Verification items for this drawing (mm, ordinates from the low corner). A direction names the side the tool comes from. Coordinates: 2 decimals unless noted, no trailing zeros. Loops run counter-clockwise (first coordinate to the right, second up) from the corner with the lowest first, then second, coordinate; pieces in that order, holes last. Notation, with made-up numbers: M 50,57.25 L 61,57.25 A12 cw 61,72.25 Z; hole C 54,12.5 d4. An arc over 180 degrees is marked long. Use CSV: the item, a comma, the result in double quotes.
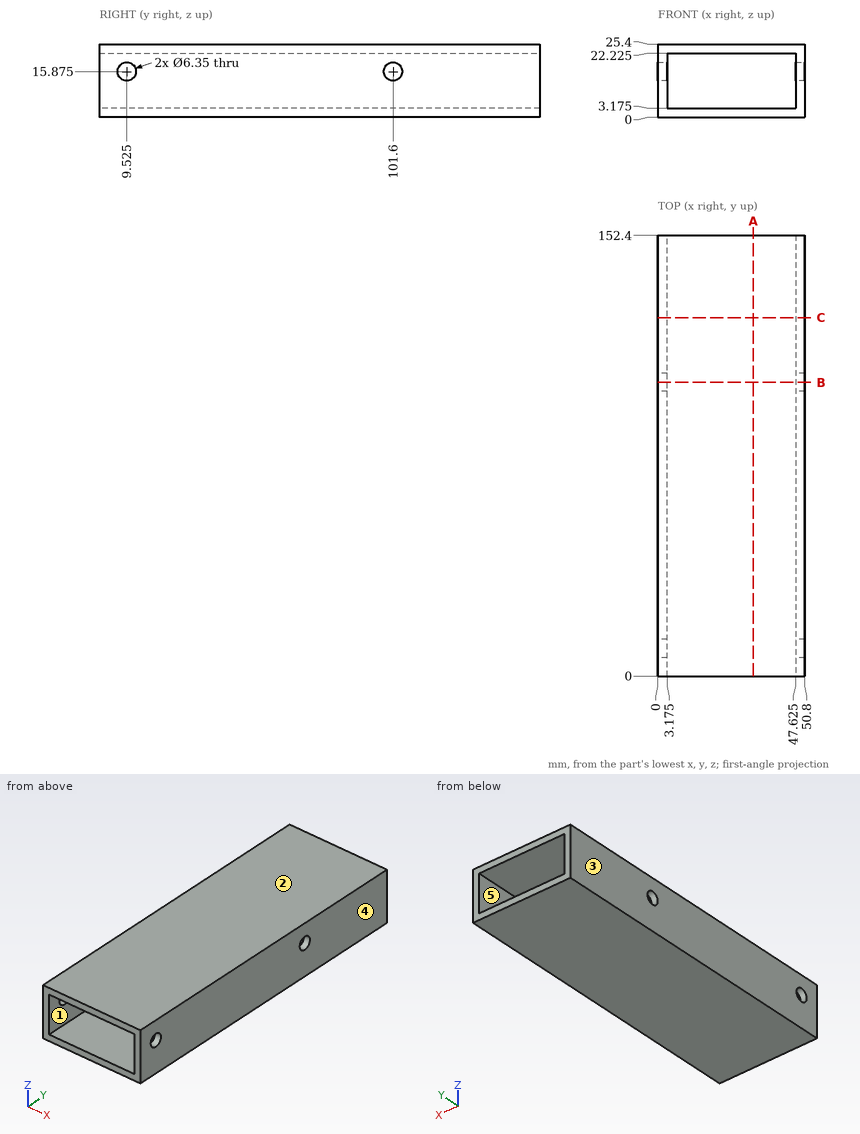
1. Set-up check for the marked faces 1 and 2: record each of +Z, -Z, +X, -X, +Y, -Y from which the full face is reachable in a straight line by a thin tool's end or side.
The answers:
face 1,"+Y, -Y"
face 2,"+Z, +X, -X, +Y, -Y"
2. Section check C-C, the plane y = 124. Record the cut outline in (x, z) (3 decimals).
The answers:
outline,"M 0,0 L 50.8,0 L 50.8,25.4 L 0,25.4 Z; hole M 3.175,3.175 L 47.625,3.175 L 47.625,22.225 L 3.175,22.225 Z"
3. Thickness scan on line 1 (X direction, y = 15, z = 21) (3 decimals); line 2 (Z direction, x = 8, y = 132) (3 decimals); line 3 (Y direction, x = 49.5, z = 13.5). Record the ranges inside material, lowest first. Write a range as [from, to].
The answers:
line 1,"[0, 3.175], [47.625, 50.8]"
line 2,"[0, 3.175], [22.225, 25.4]"
line 3,"[0, 7.42], [11.63, 99.49], [103.71, 152.4]"
4. Section check A-A, the plane x = 33. Record the cut outline in (y, z) (3 decimals), plus the area to 3 significant figures.
The answers:
outline,"M 0,0 L 152.4,0 L 152.4,3.175 L 0,3.175 Z; M 0,22.225 L 152.4,22.225 L 152.4,25.4 L 0,25.4 Z"
area,"968 mm^2"
5. Section check B-B, the plane y = 101.6. Record the cut outline in (x, z) (3 decimals).
The answers:
outline,"M 0,0 L 50.8,0 L 50.8,12.7 L 47.625,12.7 L 47.625,3.175 L 3.175,3.175 L 3.175,12.7 L 0,12.7 Z; M 0,19.05 L 3.175,19.05 L 3.175,22.225 L 47.625,22.225 L 47.625,19.05 L 50.8,19.05 L 50.8,25.4 L 0,25.4 Z"
6. Release check for a two-part mould opening along X. For the marked faces 3, 4 and 5 record: +X half, -X half, draft (parallel to the pull), parting line (faces both ways), or undercut.
The answers:
face 3,"-X half"
face 4,"+X half"
face 5,"undercut"
